Here's the drawing with two shaded views (mm, measured from the low corner). I have some questions. A direction names the side the tool comes from. Coordinates: 2 decimals unless noted, no trailing zeros. Write each loop counter-clockwise with the first axis right and the second up, starting at its lowest first coordinate (ties: lowest second). Pieces come first, ordered by that corner, then holes.
Item 1: If we section it at A-A (z = 21.5): Count the separate pieces of the cut face and the enclosed holes in it, then the cut area to 3 significant figures.
Item 2: If I drill on line 1 (Y direction, x = 75, z = 14.5); line 2 (Y direction, x = 45, z = 15.5); line 3 (X direction, y = 28.5, z = 21.5), over which ranges is the centre line in solid material (lowest first)?
Item 3: I'm going to push flat-ended pins straight in: pin 1 Ø1.5 at (x, y) = (32.5, 3) entering from -Z; pin 2 Ø3 at (x, y) = (37.5, 25) entering from -Z; pin 3 Ø8 at (x, y) = (3, 23) entering from +Z. Where does each tip first touch, or does it pass through?
Item 4: If we section it at C-C (x = 57.5): Please give me the cut outline in (y, z).
Item 5: For the marked faces 5, 6, 7, 8 and 9, which set-ups out of +Z, -Z, +X, -X, +Y, -Y let a thin tool reach every point of the face, with its end or its side?
Item 6: If we section it at D-D (z = 6.5): Please give me the cut outline in (x, y).
Item 7: We'd pull the mould along X, two halves only. Please class the marked faces 1, 2, 3 and 4: +X half, -X half, draft (parallel to the pull), parting line (faces both ways), or undercut.
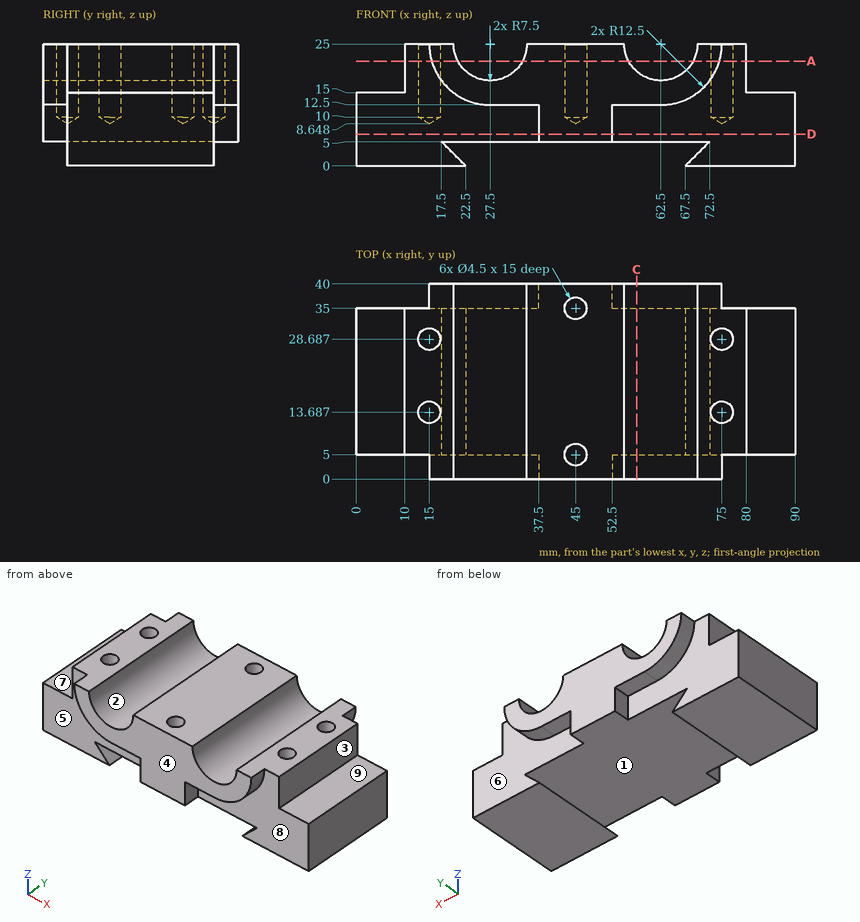
Answer list:
1. separate pieces: 3
1. enclosed holes: 6
1. area: 1,530 mm2
2. line 1: y = 5 to 11.44, 15.94 to 26.44, 30.94 to 35
2. line 2: y = 0 to 2.75, 7.25 to 32.75, 37.25 to 40
2. line 3: x = 10 to 12.76, 17.24 to 20.87, 34.13 to 55.87, 69.13 to 72.76, 77.24 to 80
3. pin 1: stops at z = 12.5
3. pin 2: stops at z = 5
3. pin 3: stops at z = 15
4. outline: (0, 12.5) - (5, 12.5) - (5, 5) - (35, 5) - (35, 12.5) - (40, 12.5) - (40, 19.41) - (0, 19.41) - close
5. face 5: -Z, -X, -Y
5. face 6: -Z, +X, +Y
5. face 7: +Z, -X, +Y, -Y
5. face 8: -Z, +X, -Y
5. face 9: +Z, +X, +Y, -Y
6. outline: (0, 5) - (37.5, 5) - (37.5, 0) - (52.5, 0) - (52.5, 5) - (90, 5) - (90, 35) - (52.5, 35) - (52.5, 40) - (37.5, 40) - (37.5, 35) - (0, 35) - close
7. face 1: undercut
7. face 2: undercut
7. face 3: +X half
7. face 4: draft
